Geometry check sheet. Reference: the model listing, model coordinates, mm. A direction names the side the tool comes from. Give positions to 0.01 mm unless a question says otherwise; leave off trailing zeros. Write each loop counter-clockwise with the first axis right and the second up, starting at its lowest first coordinate (ties: lowest second). Pieces come first, ordered by that corner, then holes.
(1) Cross-section at C-C (x = -5.5). Record the boundary of the cut face in (y, z), and give its area (3 significant figures).
(2) Cross-section at D-D (z = 21). Record the boundary of the cut face in (x, y), and give its area (3 significant figures).
(3) Mould release check, pull along Y, two halves, no side actions. Record for faces 4 (the cylindrical face through (11.605, -8.075, 35.394)), 5 (the flat face through (0, 0, 59)), 6 (the cylindrical face through (-2.17, -9.76, 41.46)): +Y half, -Y half, draft (parallel to the pull), parting line (faces both ways), or undercut.
(4) Thickness scan on line 1 along Y through (x, z) = (0, 35); line 2 along X through (y, z) = (-7.5, 35.5); line 3 along X through (y, z) = (-7, 36) (3 decimals). Record the ranges inside material, lowest first.
(5) Depth check by flat-ended pin: P1, Ø4, axis at y = -6, z = 35, coming from the +X side; P2, Ø4, axis at x = 0, y = 15, coming from the +Z side; P3, Ø0.5, axis at x = 0, y = 2.5, coming from the +Z side. Enter the tip coordinate at first touch or a pass-through.
(6) Cross-section at A-A (y = 0). Record the boundary of the cut face in (x, z), and give its area (3 significant figures).
(7) Cross-section at B-B (z = 34.5). Record the boundary of the cut face in (x, y), and give its area (3 significant figures).
(8) Tool access check on faces 1 (the cylindrical face through (1.384, -2.662, 51.395)), 2 (the flat face through (0, 2, 54)), 3 (the flat face through (0, 0, 0)). Record the directions out of +Z, -Z, +X, -X, +Y, -Y that give a thin tool (end or side, any length) a straight path to the whole face; none if there is none.
```python
from build123d import *

# Parameters (mm, degrees)
F0_R          = 20
F0_R_2        = 10
F1_DEPTH      = 39
F2_DEPTH      = 44
F3_DEPTH      = 59
F4_DEPTH      = 49
F6_R          = 4
F7_DEPTH      = 7.5
F7_DEPTH_BACK = 25.4
F8_SIZE       = 1.27
F10_D         = 3
F10_DEPTH     = 7.112
F10_TIP       = 0.9012909285


with BuildPart() as f1:
    # F0 (on Top) → F1 (new body)
    with BuildSketch(Plane.XY):
        Circle(F0_R)
        Circle(F0_R_2, mode=Mode.SUBTRACT)
    extrude(amount=F1_DEPTH)

    # F0 (on Top) → F2 (join)
    with BuildSketch(Plane.XY):
        Circle(F0_R_2)
        with BuildLine():
            ThreePointArc((2.2360679775, 2), (2.8025170769, 1.0704662693), (3, 0))
            ThreePointArc((3, 0), (-1.0704662693, -2.8025170769), (-2.2360679775, 2))
            ThreePointArc((-2.2360679775, 2), (0, 3), (2.2360679775, 2))
        make_face(mode=Mode.SUBTRACT)
    extrude(amount=F2_DEPTH)

    # F0 (on Top) → F3 (join)
    with BuildSketch(Plane.XY):
        with BuildLine():
            ThreePointArc((-2.2360679775, 2), (-1.0704662693, -2.8025170769), (3, 0))
            ThreePointArc((3, 0), (2.8025170769, 1.0704662693), (2.2360679775, 2))
            Line((2.2360679775, 2), (-2.2360679775, 2))
        make_face()
    extrude(amount=F3_DEPTH)

    # F0 (on Top) → F4 (join)
    with BuildSketch(Plane.XY):
        with BuildLine():
            Line((-2.2360679775, 2), (2.2360679775, 2))
            ThreePointArc((2.2360679775, 2), (0, 3), (-2.2360679775, 2))
        make_face()
    extrude(amount=F4_DEPTH)

    # F6 (on offset) → F7 (join, two sides)
    with BuildSketch(Plane.XZ.offset(20)) as f7_sk:
        with Locations((0, 8)):
            Circle(F6_R)
    extrude(amount=F7_DEPTH)
    extrude(f7_sk.sketch, amount=-F7_DEPTH_BACK)

    # F8
    f8_edges = [f1.edges().sort_by_distance(p)[0] for p in [
        (-4, -27.5, 8),
    ]]
    chamfer(f8_edges, length=F8_SIZE)

    # F10
    with Locations(Plane.XY.offset(39)):
        with Locations((0, 15), (-12.9903810568, -7.5), (12.9903810568, -7.5)):
            Hole(F10_D / 2, depth=F10_DEPTH)
            with Locations((0, 0, -(F10_DEPTH + F10_TIP / 2))):  # 118° drill point
                Cone(0, F10_D / 2, F10_TIP, mode=Mode.SUBTRACT)


solid = f1.part
```
Reply:
1. outline: (-19.23, 0) - (19.23, 0) - (19.23, 39) - (8.35, 39) - (8.35, 44) - (-8.35, 44) - (-8.35, 39) - (-19.23, 39) - close
1. area: 1,580 mm2
2. outline: circle Ø40 at (0, 0)
2. area: 1,260 mm2
3. face 4: undercut
3. face 5: draft
3. face 6: parting line
4. line 1: y = -20 to 13.5, 16.5 to 20
4. line 2: x = -18.54 to -14.49, -11.49 to 11.49, 14.49 to 18.54
4. line 3: x = -18.735 to -14.405, -11.576 to 11.576, 14.405 to 18.735
5. P1: stops at x = 19.6
5. P2: stops at z = 39
5. P3: stops at z = 49
6. outline: (-20, 0) - (20, 0) - (20, 39) - (10, 39) - (10, 44) - (3, 44) - (3, 59) - (-3, 59) - (-3, 44) - (-10, 44) - (-10, 39) - (-20, 39) - close
6. area: 1,750 mm2
7. outline: circle Ø40 at (0, 0); hole circle Ø3 at (-12.99, -7.5); hole circle Ø3 at (0, 15); hole circle Ø3 at (12.99, -7.5)
7. area: 1,240 mm2
8. face 1: +Z
8. face 2: +Z, +X, -X, +Y
8. face 3: -Z, +X, -X, +Y, -Y
